Read the model definition and answer for the solid it produces. Units are mm, in the model's axes. A direction names the side the tool comes from. Round coordinates to 2 decimals unless told otherwise and drop trailing zeros. Order: outer loops, then holes, each group sorted by start corner. A loop starts at its lowest first (then second) coordinate and runs counter-clockwise, first axis right, second up. Notation, with made-up numbers: (43, 74) -> (53, 74) arc R23 cw to (53, 108) -> close; hole circle Ø1 at (16, -3.75). An arc over 180 degrees is marked (long way). One line per item, written item: value. Start each with the question number.
1. Section B-B (y = 71.5) is taken. Give the vertices of the cut face in (x, z), then the cut area to 3 significant figures.
2. Section C-C (x = 124) is taken. Give the vertices of the cut face in (y, z), then the cut area to 3 significant figures.
3. For faces 1 (the face through (71, 61, 100)), 2 (the face through (69, 110, 110)), determine the directions among +Z, -Z, +X, -X, +Y, -Y from which every point of the face is accessible in a straight line to the end or side of a thin tool.
4. Consider line 1 (Z direction, x = 125, y = 16.5); line 2 (Y direction, x = 40.5, z = 17); line 3 (X direction, y = 68, z = 109.5). Determine where each line is inside the solid, lowest interval first.
5. Section A-A (x = 76) is taken. Give the vertices of the cut face in (y, z).
6. Section D-D (z = 112.5) is taken. Give the vertices of the cut face in (x, y).
7. Flat-ended cylindrical pins translate along their axes: pin 1 Ø5 at (x, y) = (88.5, 63.5) entering from -Z; pin 2 Ø12 at (x, z) = (48, 50.5) entering from +Y. Find the tip coordinate at first contact, or state that the pin passes through.
8. The mould has two halves that part along Y. Classify faces 3 (the face through (71, 9.948, 51)), 4 (the face through (69, 0, 59)), 5 (the face through (70.235, 62.738, 109.86)), 6 (the face through (0, 34, 104)): released by +Y, released by -Y, zero draft, split by the parting line, or undercut.
from build123d import *

# Parameters (mm, degrees)
SKETCH1_W               = 140
SKETCH1_H               = 110
BOSS_EXTRUDE1_DEPTH     = 120
CUT_EXTRUDE1_DEPTH      = 215.709105536
CUT_EXTRUDE1_DEPTH_BACK = 100
SKETCH3_R               = 15.739400913
CUT_EXTRUDE2_DEPTH      = 205.205778567


with BuildPart() as part:
    # Sketch1 → Boss-Extrude1 (new body)
    with BuildSketch(Plane.XY):
        with Locations((70, 55)):
            Rectangle(SKETCH1_W, SKETCH1_H)
    extrude(amount=BOSS_EXTRUDE1_DEPTH)

    # Sketch2 → Cut-Extrude1 (cut, two sides: drawn at the far end of the back side and taken through both)
    with BuildSketch(Plane(origin=(0, 0, 0), x_dir=(-1, 0, 0), z_dir=(0, 0, -1)).offset(-CUT_EXTRUDE1_DEPTH_BACK)):
        Polygon((-494.154006157, 9.947538818), (-140, 9.947538818), (0, 9.947538818), (354.154006157, 9.947538818), (354.154006157, 718.255551133), (-494.154006157, 718.255551133), align=None)
    extrude(amount=CUT_EXTRUDE1_DEPTH + CUT_EXTRUDE1_DEPTH_BACK, mode=Mode.SUBTRACT)

    # Sketch3 → Cut-Extrude2 (cut, through all)
    with BuildSketch(Plane(origin=(0, 0, 100), x_dir=(-1, 0, 0), z_dir=(0, 0, -1))):
        with Locations((-77.497780525, 76.701563568)):
            Circle(SKETCH3_R)
    extrude(amount=-CUT_EXTRUDE2_DEPTH, mode=Mode.SUBTRACT)


solid = part.part
Answer:
1. outline: (0, 100) -> (62.64, 100) -> (62.64, 120) -> (0, 120) -> close; (92.35, 100) -> (140, 100) -> (140, 120) -> (92.35, 120) -> close
1. area: 2,210 mm^2
2. outline: (0, 0) -> (9.95, 0) -> (9.95, 100) -> (110, 100) -> (110, 120) -> (0, 120) -> close
2. area: 3,190 mm^2
3. face 1: -Z, +X, -X, +Y
3. face 2: +Z, -Z, +X, -X, +Y
4. line 1: 100 to 120
4. line 2: 0 to 9.95
4. line 3: 0 to 64.38, 90.61 to 140
5. outline: (0, 0) -> (9.95, 0) -> (9.95, 100) -> (61.03, 100) -> (61.03, 120) -> (0, 120) -> close; (92.37, 100) -> (110, 100) -> (110, 120) -> (92.37, 120) -> close
6. outline: (0, 0) -> (140, 0) -> (140, 110) -> (0, 110) -> close; hole circle Ø31.48 at (77.5, 76.7)
7. pin 1: z = 100
7. pin 2: y = 9.95
8. face 3: released by +Y
8. face 4: released by -Y
8. face 5: undercut
8. face 6: zero draft
